Part model, mm, in its own coordinate system. Face numbers are marked on the shaded views. A direction names the side the tool comes from. Coordinates: 2 decimals unless noted, no trailing zeros. Order: outer loops, then holes, each group sorted by start corner. A loop starts at its lowest first (then second) coordinate and runs counter-clockwise, first axis right, second up. Notation, with made-up numbers: (3, 25.5) - (31, 25.5) arc R24 cw to (31, 50.5) - close; hole circle Ø6 at (2, -24). An arc over 180 degrees is marked (long way). Use a Markdown table: item, result. Add a question column.
1) Saw through at C-C on z = 12. List the corners of the cut face in (x, y), then the cut area to 3 significant figures.
2) Drop flat-ended pins along their axis: P1, Ø3, axis at x = 14.5, y = -9.5, coming from the +Z side; P2, Ø4.5, axis at x = -100, z = -57, coming from the -Y side; P3, Ø3.5, axis at x = -48, z = -17.5, coming from the -Y side. Give the stop position or say it passes through.
3) Saw through at B-B on x = -73.5. List the corners of the cut face in (y, z), then the cut area to 3 significant figures.
4) Wall check: L1, parallel to X at y = -14, z = 57; L2, parallel to X at y = -20, z = -24; L3, parallel to Z at x = 97.5, y = -22.5. Give the ranges that are in metal, low to high. Write a range as [from, to].
5) Two-plate mould, pull along X, no slides. Class the marked faces 1, 2 and 3: +X half, -X half, draft (parallel to the pull), parting line (faces both ways), or undercut.
6) Saw through at A-A on y = -18.5. Count the separate pieces of the cut face and the enclosed holes in it, then the cut area to 3 significant figures.
7) Tool access for the marked faces 4 and 5: list every direction of +Z, -Z, +X, -X, +Y, -Y with a clear straight run to the whole face (end or side of a thin tool).
```python
from build123d import *

# Parameters (mm, degrees)
SKETCH_1_W                     = 220
SKETCH_1_H                     = 135
BASE_FLOOR_3MM_DEPTH           = 3
SKETCH_2_W                     = 220
SKETCH_2_H                     = 3
BACK_WALL_DEPTH                = 37
SKETCH_3_W                     = 3
SKETCH_3_H                     = 132
LEFT_WALL_DEPTH                = 37
SKETCH_4_W                     = 3
SKETCH_4_H                     = 132
RIGHT_WALL_DEPTH               = 37
SKETCH_5_W                     = 32
SKETCH_5_H                     = 3
FRONT_LEFT_WALL_DEPTH          = 37
SKETCH_6_W                     = 30
SKETCH_6_H                     = 3
FRONT_CAMERA_BRIDGE_DEPTH      = 37
SKETCH_7_W                     = 59
SKETCH_7_H                     = 3
FRONT_SR04_BRIDGE_DEPTH        = 37
SKETCH_8_W                     = 18
SKETCH_8_H                     = 3
FRONT_RIGHT_WALL_DEPTH         = 37
SKETCH_9_R                     = 5
LID_BOSS_1_DEPTH               = 30
SKETCH_10_R                    = 1.35
LID_BOSS_1_PILOT_DEPTH         = 34
SKETCH_11_R                    = 5
LID_BOSS_2_DEPTH               = 30
SKETCH_12_R                    = 1.35
LID_BOSS_2_PILOT_DEPTH         = 34
SKETCH_13_R                    = 5
LID_BOSS_3_DEPTH               = 30
SKETCH_14_R                    = 1.35
LID_BOSS_3_PILOT_DEPTH         = 34
SKETCH_15_R                    = 5
LID_BOSS_4_DEPTH               = 30
SKETCH_16_R                    = 1.35
LID_BOSS_4_PILOT_DEPTH         = 34
SKETCH_17_R                    = 1.6
P4_NANO_PEG_1_DEPTH            = 7
SKETCH_18_R                    = 1.6
P4_NANO_PEG_2_DEPTH            = 7
SKETCH_19_R                    = 1.6
P4_NANO_PEG_3_DEPTH            = 7
SKETCH_20_R                    = 1.6
P4_NANO_PEG_4_DEPTH            = 7
SKETCH_21_R                    = 1.6
MEGA_PEG_1_DEPTH               = 7
SKETCH_22_R                    = 1.6
MEGA_PEG_2_DEPTH               = 7
SKETCH_23_R                    = 1.6
MEGA_PEG_3_DEPTH               = 7
SKETCH_24_R                    = 1.6
MEGA_PEG_4_DEPTH               = 7
SKETCH_25_W                    = 12
SKETCH_25_H                    = 3.4
CABLE_TIE_SLOT_1_DEPTH         = 4
SKETCH_26_W                    = 12
SKETCH_26_H                    = 3.4
CABLE_TIE_SLOT_2_DEPTH         = 4
SKETCH_27_W                    = 12
SKETCH_27_H                    = 3.4
CABLE_TIE_SLOT_3_DEPTH         = 4
SKETCH_28_W                    = 12
SKETCH_28_H                    = 3.4
CABLE_TIE_SLOT_4_DEPTH         = 4
SKETCH_29_W                    = 12
SKETCH_29_H                    = 3.4
CABLE_TIE_SLOT_5_DEPTH         = 4
SKETCH_30_W                    = 12
SKETCH_30_H                    = 3.4
CABLE_TIE_SLOT_6_DEPTH         = 4
SKETCH_31_W                    = 67
SKETCH_31_H                    = 3
ADJUSTABLE_SENSOR_RAIL_1_DEPTH = 4
SKETCH_32_W                    = 67
SKETCH_32_H                    = 3
ADJUSTABLE_SENSOR_RAIL_2_DEPTH = 4


with BuildPart() as part:
    # 草图1 → Base_Floor_3mm (new body)
    with BuildSketch(Plane(origin=(0, 0, 0), x_dir=(1, 0, 0), z_dir=(0, 1, 0))):
        Rectangle(SKETCH_1_W, SKETCH_1_H)
    extrude(amount=-BASE_FLOOR_3MM_DEPTH)

    # 草图2 → Back_Wall (add)
    with BuildSketch(Plane(origin=(0, 0, 0), x_dir=(1, 0, 0), z_dir=(0, 1, 0))):
        with Locations((0, 66)):
            Rectangle(SKETCH_2_W, SKETCH_2_H)
    extrude(amount=-BACK_WALL_DEPTH)

    # 草图3 → Left_Wall (add)
    with BuildSketch(Plane(origin=(0, 0, 0), x_dir=(1, 0, 0), z_dir=(0, 1, 0))):
        with Locations((-108.5, -1.5)):
            Rectangle(SKETCH_3_W, SKETCH_3_H)
    extrude(amount=-LEFT_WALL_DEPTH)

    # 草图4 → Right_Wall (add)
    with BuildSketch(Plane(origin=(0, 0, 0), x_dir=(1, 0, 0), z_dir=(0, 1, 0))):
        with Locations((108.5, -1.5)):
            Rectangle(SKETCH_4_W, SKETCH_4_H)
    extrude(amount=-RIGHT_WALL_DEPTH)

    # 草图5 → Front_Left_Wall (add)
    with BuildSketch(Plane(origin=(0, 0, 0), x_dir=(1, 0, 0), z_dir=(0, 1, 0))):
        with Locations((-94, -66)):
            Rectangle(SKETCH_5_W, SKETCH_5_H)
    extrude(amount=-FRONT_LEFT_WALL_DEPTH)

    # 草图6 → Front_Camera_Bridge (add)
    with BuildSketch(Plane(origin=(0, 0, 0), x_dir=(1, 0, 0), z_dir=(0, 1, 0))):
        with Locations((-27, -66)):
            Rectangle(SKETCH_6_W, SKETCH_6_H)
    extrude(amount=-FRONT_CAMERA_BRIDGE_DEPTH)

    # 草图7 → Front_SR04_Bridge (add)
    with BuildSketch(Plane(origin=(0, 0, 0), x_dir=(1, 0, 0), z_dir=(0, 1, 0))):
        with Locations((47.5, -66)):
            Rectangle(SKETCH_7_W, SKETCH_7_H)
    extrude(amount=-FRONT_SR04_BRIDGE_DEPTH)

    # 草图8 → Front_Right_Wall (add)
    with BuildSketch(Plane(origin=(0, 0, 0), x_dir=(1, 0, 0), z_dir=(0, 1, 0))):
        with Locations((101, -66)):
            Rectangle(SKETCH_8_W, SKETCH_8_H)
    extrude(amount=-FRONT_RIGHT_WALL_DEPTH)

    # 草图9 → Lid_Boss_1 (add)
    with BuildSketch(Plane(origin=(0, 0, 0), x_dir=(1, 0, 0), z_dir=(0, 1, 0))):
        with Locations(Location((-100, -57, 0), (0, 0, 270))):
            Circle(SKETCH_9_R)
    extrude(amount=-LID_BOSS_1_DEPTH)

    # 草图10 → Lid_Boss_1_Pilot (cut)
    with BuildSketch(Plane(origin=(0, 0, 0), x_dir=(1, 0, 0), z_dir=(0, 1, 0))):
        with Locations(Location((-100, -57, 0), (0, 0, 270))):
            Circle(SKETCH_10_R)
    extrude(amount=-LID_BOSS_1_PILOT_DEPTH, mode=Mode.SUBTRACT)

    # 草图11 → Lid_Boss_2 (add)
    with BuildSketch(Plane(origin=(0, 0, 0), x_dir=(1, 0, 0), z_dir=(0, 1, 0))):
        with Locations(Location((100, -57, 0), (0, 0, 270))):
            Circle(SKETCH_11_R)
    extrude(amount=-LID_BOSS_2_DEPTH)

    # 草图12 → Lid_Boss_2_Pilot (cut)
    with BuildSketch(Plane(origin=(0, 0, 0), x_dir=(1, 0, 0), z_dir=(0, 1, 0))):
        with Locations(Location((100, -57, 0), (0, 0, 270))):
            Circle(SKETCH_12_R)
    extrude(amount=-LID_BOSS_2_PILOT_DEPTH, mode=Mode.SUBTRACT)

    # 草图13 → Lid_Boss_3 (add)
    with BuildSketch(Plane(origin=(0, 0, 0), x_dir=(1, 0, 0), z_dir=(0, 1, 0))):
        with Locations(Location((-100, 57, 0), (0, 0, 270))):
            Circle(SKETCH_13_R)
    extrude(amount=-LID_BOSS_3_DEPTH)

    # 草图14 → Lid_Boss_3_Pilot (cut)
    with BuildSketch(Plane(origin=(0, 0, 0), x_dir=(1, 0, 0), z_dir=(0, 1, 0))):
        with Locations(Location((-100, 57, 0), (0, 0, 270))):
            Circle(SKETCH_14_R)
    extrude(amount=-LID_BOSS_3_PILOT_DEPTH, mode=Mode.SUBTRACT)

    # 草图15 → Lid_Boss_4 (add)
    with BuildSketch(Plane(origin=(0, 0, 0), x_dir=(1, 0, 0), z_dir=(0, 1, 0))):
        with Locations(Location((100, 57, 0), (0, 0, 270))):
            Circle(SKETCH_15_R)
    extrude(amount=-LID_BOSS_4_DEPTH)

    # 草图16 → Lid_Boss_4_Pilot (cut)
    with BuildSketch(Plane(origin=(0, 0, 0), x_dir=(1, 0, 0), z_dir=(0, 1, 0))):
        with Locations(Location((100, 57, 0), (0, 0, 270))):
            Circle(SKETCH_16_R)
    extrude(amount=-LID_BOSS_4_PILOT_DEPTH, mode=Mode.SUBTRACT)

    # 草图17 → P4_NANO_Peg_1 (add)
    with BuildSketch(Plane(origin=(0, 0, 0), x_dir=(1, 0, 0), z_dir=(0, 1, 0))):
        with Locations(Location((-93, 18, 0), (0, 0, 270))):
            Circle(SKETCH_17_R)
    extrude(amount=-P4_NANO_PEG_1_DEPTH)

    # 草图18 → P4_NANO_Peg_2 (add)
    with BuildSketch(Plane(origin=(0, 0, 0), x_dir=(1, 0, 0), z_dir=(0, 1, 0))):
        with Locations(Location((-48, 18, 0), (0, 0, 270))):
            Circle(SKETCH_18_R)
    extrude(amount=-P4_NANO_PEG_2_DEPTH)

    # 草图19 → P4_NANO_Peg_3 (add)
    with BuildSketch(Plane(origin=(0, 0, 0), x_dir=(1, 0, 0), z_dir=(0, 1, 0))):
        with Locations((-93, 63)):
            Circle(SKETCH_19_R)
    extrude(amount=-P4_NANO_PEG_3_DEPTH)

    # 草图20 → P4_NANO_Peg_4 (add)
    with BuildSketch(Plane(origin=(0, 0, 0), x_dir=(1, 0, 0), z_dir=(0, 1, 0))):
        with Locations((-48, 63)):
            Circle(SKETCH_20_R)
    extrude(amount=-P4_NANO_PEG_4_DEPTH)

    # 草图21 → Mega_Peg_1 (add)
    with BuildSketch(Plane(origin=(0, 0, 0), x_dir=(1, 0, 0), z_dir=(0, 1, 0))):
        with Locations(Location((0, -30, 0), (0, 0, 270))):
            Circle(SKETCH_21_R)
    extrude(amount=-MEGA_PEG_1_DEPTH)

    # 草图22 → Mega_Peg_2 (add)
    with BuildSketch(Plane(origin=(0, 0, 0), x_dir=(1, 0, 0), z_dir=(0, 1, 0))):
        with Locations(Location((96, -30, 0), (0, 0, 270))):
            Circle(SKETCH_22_R)
    extrude(amount=-MEGA_PEG_2_DEPTH)

    # 草图23 → Mega_Peg_3 (add)
    with BuildSketch(Plane(origin=(0, 0, 0), x_dir=(1, 0, 0), z_dir=(0, 1, 0))):
        with Locations(Location((0, 12, 0), (0, 0, 270))):
            Circle(SKETCH_23_R)
    extrude(amount=-MEGA_PEG_3_DEPTH)

    # 草图24 → Mega_Peg_4 (add)
    with BuildSketch(Plane(origin=(0, 0, 0), x_dir=(1, 0, 0), z_dir=(0, 1, 0))):
        with Locations(Location((96, 12, 0), (0, 0, 270))):
            Circle(SKETCH_24_R)
    extrude(amount=-MEGA_PEG_4_DEPTH)

    # 草图25 → Cable_Tie_Slot_1 (cut)
    with BuildSketch(Plane(origin=(0, 0, 0), x_dir=(1, 0, 0), z_dir=(0, 1, 0))):
        with Locations((-74, 6)):
            Rectangle(SKETCH_25_W, SKETCH_25_H)
    extrude(amount=-CABLE_TIE_SLOT_1_DEPTH, mode=Mode.SUBTRACT)

    # 草图26 → Cable_Tie_Slot_2 (cut)
    with BuildSketch(Plane(origin=(0, 0, 0), x_dir=(1, 0, 0), z_dir=(0, 1, 0))):
        with Locations((-28, 6)):
            Rectangle(SKETCH_26_W, SKETCH_26_H)
    extrude(amount=-CABLE_TIE_SLOT_2_DEPTH, mode=Mode.SUBTRACT)

    # 草图27 → Cable_Tie_Slot_3 (cut)
    with BuildSketch(Plane(origin=(0, 0, 0), x_dir=(1, 0, 0), z_dir=(0, 1, 0))):
        with Locations((-5, -45)):
            Rectangle(SKETCH_27_W, SKETCH_27_H)
    extrude(amount=-CABLE_TIE_SLOT_3_DEPTH, mode=Mode.SUBTRACT)

    # 草图28 → Cable_Tie_Slot_4 (cut)
    with BuildSketch(Plane(origin=(0, 0, 0), x_dir=(1, 0, 0), z_dir=(0, 1, 0))):
        with Locations((36, -45)):
            Rectangle(SKETCH_28_W, SKETCH_28_H)
    extrude(amount=-CABLE_TIE_SLOT_4_DEPTH, mode=Mode.SUBTRACT)

    # 草图29 → Cable_Tie_Slot_5 (cut)
    with BuildSketch(Plane(origin=(0, 0, 0), x_dir=(1, 0, 0), z_dir=(0, 1, 0))):
        with Locations((75, -45)):
            Rectangle(SKETCH_29_W, SKETCH_29_H)
    extrude(amount=-CABLE_TIE_SLOT_5_DEPTH, mode=Mode.SUBTRACT)

    # 草图30 → Cable_Tie_Slot_6 (cut)
    with BuildSketch(Plane(origin=(0, 0, 0), x_dir=(1, 0, 0), z_dir=(0, 1, 0))):
        with Locations((75, 28)):
            Rectangle(SKETCH_30_W, SKETCH_30_H)
    extrude(amount=-CABLE_TIE_SLOT_6_DEPTH, mode=Mode.SUBTRACT)

    # 草图31 → Adjustable_Sensor_Rail_1 (add)
    with BuildSketch(Plane(origin=(0, 0, 0), x_dir=(1, 0, 0), z_dir=(0, 1, 0))):
        with Locations((61.5, 32.5)):
            Rectangle(SKETCH_31_W, SKETCH_31_H)
    extrude(amount=-ADJUSTABLE_SENSOR_RAIL_1_DEPTH)

    # 草图32 → Adjustable_Sensor_Rail_2 (add)
    with BuildSketch(Plane(origin=(0, 0, 0), x_dir=(1, 0, 0), z_dir=(0, 1, 0))):
        with Locations((61.5, 50.5)):
            Rectangle(SKETCH_32_W, SKETCH_32_H)
    extrude(amount=-ADJUSTABLE_SENSOR_RAIL_2_DEPTH)


solid = part.part
```
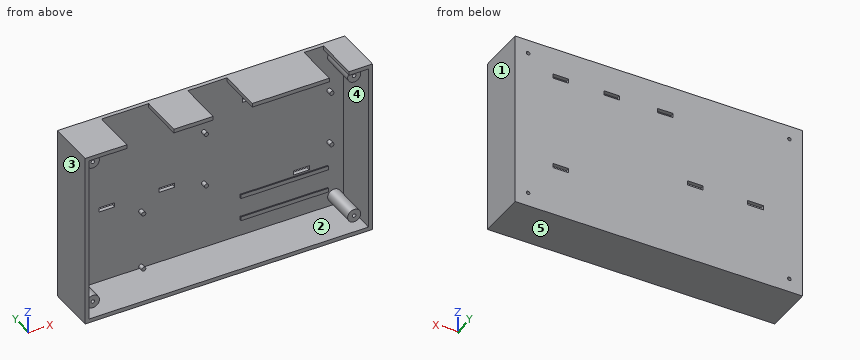
Results are:
| question | item | result |
|---|---|---|
| 1 | outline | (-110, -37) - (-107, -37) - (-107, -3) - (107, -3) - (107, -37) - (110, -37) - (110, 0) - (-110, 0) - close |
| 1 | area | 864 mm2 |
| 2 | P1 | z = -64.5 |
| 2 | P2 | y = -30 |
| 2 | P3 | y = -7 |
| 3 | outline | (-37, -67.5) - (0, -67.5) - (0, -7.7) - (-3, -7.7) - (-3, -64.5) - (-37, -64.5) - close; (-3, -4.3) - (0, -4.3) - (0, 67.5) - (-3, 67.5) - close |
| 3 | area | 497 mm2 |
| 4 | L1 | [-110, -107], [-105, -101.35], [-98.65, -95], [95, 98.65], [101.35, 105], [107, 110] |
| 4 | L2 | [-110, -107], [107, 110] |
| 4 | L3 | [-67.5, -64.5], [-61.33, -52.67], [52.67, 61.33], [64.5, 67.5] |
| 5 | face 1 | +X half |
| 5 | face 2 | undercut |
| 5 | face 3 | -X half |
| 6 | separate pieces | 7 |
| 6 | enclosed holes | 4 |
| 6 | area | 2,140 mm2 |
| 7 | face 4 | -Y |
| 7 | face 5 | -Z, +X, -X, +Y, -Y |
